Autodesk Inventor part; units mm, degrees
ref_plane "YZ Plane" through (0, 0, 0) normal (1, 0, 0) x (0, 1, 0)
ref_plane "XZ Plane" through (0, 0, 0) normal (0, 1, 0) x (-1, 0, 0)
ref_plane "XY Plane" through (0, 0, 0) normal (0, 0, 1) x (1, 0, 0)
sketch "Sketch1" plane through (0, 0, 0) normal (0, 0, 1) x (1, 0, 0)
  line L0 (0, 0) -> (-50, 0)
  line L1 (-50, 0) -> (-50, 2)
  line L2 (-46, 4) -> (-46, 2)
  line L3 (-46, 2) -> (-50, 2)
  line L4 (0, 2) -> (-4, 2)
  line L5 (-4, 2) -> (-4, 4)
  line L6 (-46, 4) -> (-26, 4)
  line L7 (0, 2) -> (0, 0)
  line L8 (-26, 4) -> (-26, 2)
  line L9 (-26, 2) -> (-24, 2)
  line L10 (-24, 2) -> (-24, 4)
  line L11 (-24, 4) -> (-4, 4)
  dimension "d2" = 4
  dimension "d3" = 2
  dimension "d5" = 24
  dimension "d6" = 2
  dimension "d7" = 2
extrude "Extrusion1" add sketch "Sketch1" along normal blind 2
sketch "Sketch2" plane through (0, 0, 2) normal (0, 0, 1) x (1, 0, 0)
  line L0 (-4, 4) -> (-24, 4)
  line L1 (-18, 4) -> (-16, 4)
  line L2 (-16, 4) -> (-16, 2)
  line L3 (-16, 2) -> (-18, 2)
  line L4 (-18, 2) -> (-18, 4)
  point P0 (0, 0)
  dimension "d10" = 2
  dimension "d11" = 2
  dimension "d12" = 16
extrude "Extrusion2" cut sketch "Sketch2" against normal blind 2
sketch "Sketch3" plane through (0, 0, 0) normal (0, 0, -1) x (-1, 0, 0)
  line L0 (18, 4) -> (24, 4)
  line L1 (50, 2) -> (50, 0)
  line L2 (18, 4) -> (50, 4)
  line L3 (50, 4) -> (50, 0)
  line L4 (50, 0) -> (18, 0)
  line L5 (18, 0) -> (18, 4)
  line L6 (0, 2) -> (4, 2)
  line L7 (0, 0) -> (0, 2)
  line L8 (4, 2) -> (0, 2)
  line L9 (0, 2) -> (0, 0)
  line L10 (0, 0) -> (4, 0)
  line L11 (4, 0) -> (4, 2)
  line L12 (4, 2) -> (4, 4)
  line L13 (4, 4) -> (6, 4)
  line L14 (6, 4) -> (6, 2)
  line L15 (6, 2) -> (4, 2)
  line L16 (4, 2) -> (4, 4)
  dimension "d17" = 2
extrude "Extrusion3" cut sketch "Sketch3" against normal blind 10
properties part number "beam1" material "Wood (Birch)"
Geometry: final body of the model. Coordinates: model frame, mm. A direction names the side the tool comes from. Coordinates: 2 decimals unless noted, no trailing zeros. Order: outer loops, then holes, each group sorted by start corner. A loop starts at its lowest first (then second) coordinate and runs counter-clockwise, first axis right, second up.
(1) Section query A-A (z = 0.3). Return the cut outline in (x, y), plus the area to 3 significant figures.
(2) Section query C-C (x = -16.5). Return the cut outline in (y, z).
(3) Access query for faces 1 (the face through (-11, 2, 0)), 2 (the face through (-17, 2, 1)), 3 (the face through (-5, 2, 1)). Directions: +Z, -Z, +X, -X, +Y, -Y. A direction counts if a zero-diameter tool reaches every point of the face in a straight line with its end or side. Return the directions, or none.
(4) Section query B-B (y = 3.15). Return the cut outline in (x, z), plus the area to 3 significant figures.
(5) Material intervals for probe 1 along Y at (x, z) = (-17, 1.35); probe 2 along X at (y, z) = (3.25, 1.9), sorted ascending.
Solution:
1. outline: (-18, 0) - (-4, 0) - (-4, 2) - (-6, 2) - (-6, 4) - (-16, 4) - (-16, 2) - (-18, 2) - close
1. area: 48.0 mm2
2. outline: (0, 0) - (2, 0) - (2, 2) - (0, 2) - close
3. face 1: -Z, +X, -X, +Y, -Y
3. face 2: +Z, -Z, -X, +Y
3. face 3: +Z, -Z, +X, +Y
4. outline: (-16, 0) - (-6, 0) - (-6, 2) - (-16, 2) - close
4. area: 20.0 mm2
5. probe 1: y = 0 to 2
5. probe 2: x = -16 to -6
